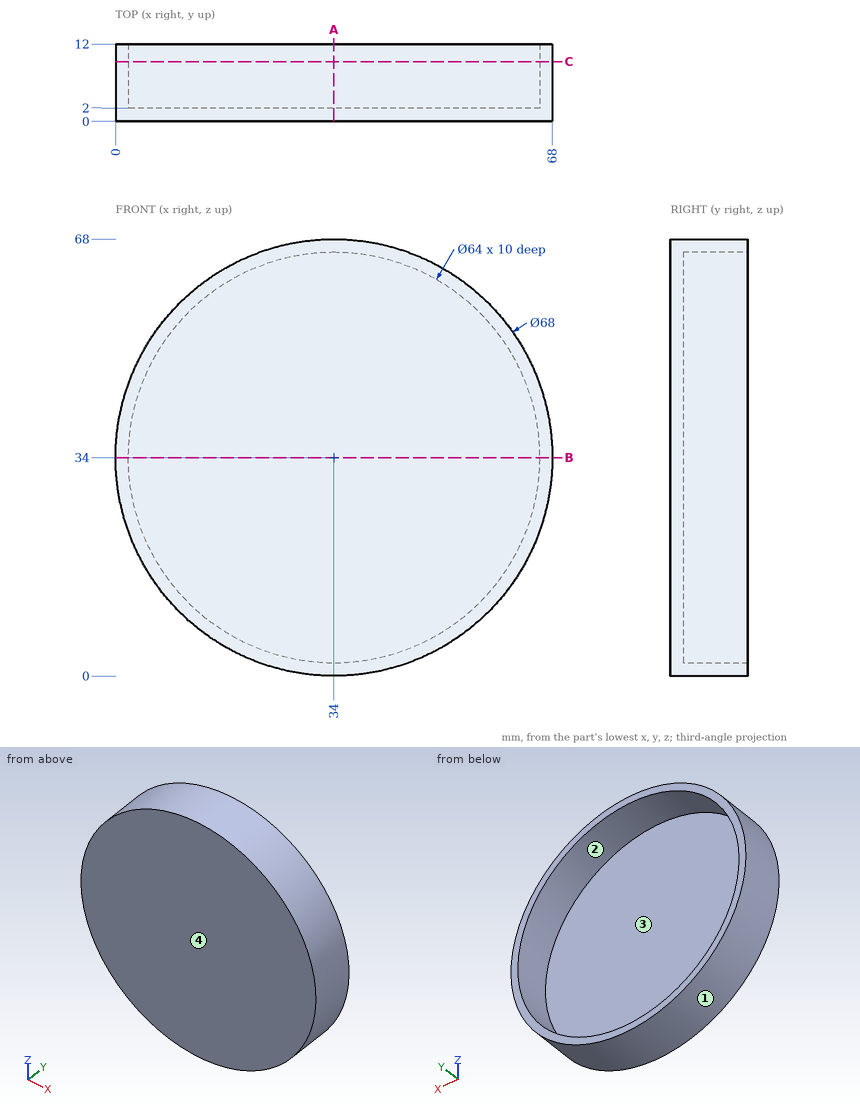
Design review of the part shown in the three views and the two pictorial views. Dimensions are in mm from the part's minimum x, y and z. Round coordinates to 2 decimals unless told otherwise and drop trailing zeros. Loops run counter-clockwise (first coordinate to the right, second up) from the corner with the lowest first, then second, coordinate; pieces in that order, holes last. Notation, with made-up numbers: (45.25, -18) - (78.25, -18) arc R25 cw to (78.25, 18) - close; hole circle Ø7 at (6, -25). An arc over 180 degrees is marked (long way). Use CSV: the item, a comma, the result in double quotes.
(1) Take a section at B-B, the plane z = 34. Give the boundary of the cut face in (x, y), plus the area to 3 significant figures.
Working result:
outline,"(0, 0) - (68, 0) - (68, 12) - (66, 12) - (66, 2) - (2, 2) - (2, 12) - (0, 12) - close"
area,"176 mm^2"
(2) For line 1 (X direction, y = 8.75, z = 34); line 2 (Y direction, x = 26.5, z = 48); line 3 (Z direction, x = 24, y = 8), list the stretches that pass through material, from the lowest coordinate up.
Working result:
line 1,"x = 0 to 2, 66 to 68"
line 2,"y = 0 to 2"
line 3,"z = 1.5 to 3.6, 64.4 to 66.5"
(3) Take a section at A-A, the plane x = 34. Give the boundary of the cut face in (y, z).
Working result:
outline,"(0, 0) - (12, 0) - (12, 2) - (2, 2) - (2, 66) - (12, 66) - (12, 68) - (0, 68) - close"
(4) The part is to be moulded in two halves that separate along Z. For the marked faces 1, 2, 3 and 4, say which applies: pulls with the +Z half, pulls with the -Z half, needs draft (parallel to the pull), parting line crosses it, or undercut.
Working result:
face 1,"parting line crosses it"
face 2,"undercut"
face 3,"undercut"
face 4,"needs draft"
(5) Take a section at C-C, the plane y = 9.25. Give the boundary of the cut face in (x, z).
Working result:
outline,"circle Ø68 at (34, 34); hole circle Ø64 at (34, 34)"
(6) Clearance check with flat-ended pins moving along their axes: P1, Ø1, axis at x = 38, y = 6.5, coming from the -Z side; P2, Ø6, axis at x = 9, y = 7.5, coming from the +Z side; P3, Ø1, axis at y = 3.5, z = 40, coming from the +X side. State where each tip first meets the part, or that it passes through.
Working result:
P1,"stops at z = 0.18"
P2,"stops at z = 59.92"
P3,"stops at x = 67.55"
